from build123d import *

# Parameters (mm, degrees)
BOSS_EXTRUDE1_DEPTH = 2


with BuildPart() as part:
    # Sketch1 → Boss-Extrude1 (new body)
    with BuildSketch(Plane(origin=(0, 0, 0), x_dir=(0, 0, -1), z_dir=(1, 0, 0))):
        Polygon((20, 0), (0, 0), (0, 25), (-20, 25), (-20, 0), (-40, 0), (-40, -70), (20, -70), align=None)
        with BuildLine():
            ThreePointArc((9.318516526, -50.176380902), (-10, -65), (-29.318516526, -50.176380902))
            Line((-29.318516526, -50.176380902), (-32.5, -45))
            Line((-32.5, -45), (-32.5, -5))
            Line((-32.5, -5), (-20, -5))
            Line((-20, -5), (-20, -25))
            Line((-20, -25), (-17.5, -25))
            Line((-17.5, -25), (-15.75, -24.318465914))
            ThreePointArc((-15.75, -24.318465914), (-10, -22.5), (-4.25, -24.318465914))
            Line((-4.25, -24.318465914), (-2.5, -25))
            Line((-2.5, -25), (0, -25))
            Line((0, -25), (0, -4.981590289))
            Line((0, -4.981590289), (12.5, -5))
            Line((12.5, -5), (12.5, -45))
            Line((12.5, -45), (9.318516526, -50.176380902))
        make_face(mode=Mode.SUBTRACT)
    extrude(amount=BOSS_EXTRUDE1_DEPTH)


solid = part.part
Geometry: final body of the model. Coordinates: model frame, mm. A direction names the side the tool comes from. Coordinates: 2 decimals unless noted, no trailing zeros. Order: outer loops, then holes, each group sorted by start corner. A loop starts at its lowest first (then second) coordinate and runs counter-clockwise, first axis right, second up. Notation, with made-up numbers: (-28, -31.75) - (-9, -31.75) arc R16 ccw to (-9, -2.75) - close; hole circle Ø11 at (54.25, -6.75). An arc over 180 degrees is marked (long way). Use one line per item in the form item = value.
1) Set-up query: faces 5 (the face through (1, 13, 20)), 6 (the face through (1, 12, 0)), 7 (the face through (1, -25, 32.5)). Return all of +Z, -Z, +X, -X, +Y, -Y with unobstructed straight access to the full face (end or side cutting, diameter ignored); none if empty.
Solutions:
face_5 = +Z, +X, -X, +Y
face_6 = -Z, +X, -X, +Y
face_7 = +X, -X
2) Section B-B (y = -37). Return loops of the section in (x, z).
Solutions:
outline = (0, -20) - (2, -20) - (2, -12.5) - (0, -12.5) - close; (0, 32.5) - (2, 32.5) - (2, 40) - (0, 40) - close
3) Section A-A (y = -14). Return loops of the section in (x, z), then the cut area to 3 significant figures.
Solutions:
outline = (0, -20) - (2, -20) - (2, -12.5) - (0, -12.5) - close; (0, 0) - (2, 0) - (2, 20) - (0, 20) - close; (0, 32.5) - (2, 32.5) - (2, 40) - (0, 40) - close
area = 70.0 mm^2
4) Pin query (flat end, axial travel): pin 1 (0.6 mm diameter, centred on x = 1.5, z = -6, fed in from +Y); pin 2 (3 mm diameter, centred on y = 7.5, z = 18.5, fed in from -X); pin 3 (1 mm diameter, centred on x = 1, y = 13, fed in from -Z). Return the tip coordinate at first contact, or that it passes through.
Solutions:
pin_1 = 0
pin_2 = 0
pin_3 = 0
5) Section C-C (z = 5.5). Return loops of the section in (x, y).
Solutions:
outline = (0, -70) - (2, -70) - (2, -64.49) - (0, -64.49) - close; (0, -23.57) - (2, -23.57) - (2, 25) - (0, 25) - close
6) Section D-D (x = 0.4). Return loops of the section in (y, z), then the cut area to 3 significant figures.
Solutions:
outline = (-70, -20) - (0, -20) - (0, 0) - (25, 0) - (25, 20) - (0, 20) - (0, 40) - (-70, 40) - close; hole (-50.18, -9.32) - (-45, -12.5) - (-5, -12.5) - (-4.98, 0) - (-25, 0) - (-25, 2.5) - (-24.32, 4.25) arc R10 ccw to (-24.32, 15.75) - (-25, 17.5) - (-25, 20) - (-5, 20) - (-5, 32.5) - (-45, 32.5) - (-50.18, 29.32) arc R20 ccw to start
area = 2,640 mm^2
7) Mould query, pull axis Y, two halves, no side actions, for faces 1 (the face through (1, -5, 26)), 2 (the face through (0, -22, 10)), 3 (the face through (1, -70, 10)), 4 (the face through (1, 25, 10)). Classes: +Y half, -Y half, draft (parallel to the pull), parting line (faces both ways), or undercut.
Solutions:
face_1 = undercut
face_2 = draft
face_3 = -Y half
face_4 = +Y half
8) Ray query, L1, parallel to Z at x = 1.35, y = -14; L2, parallel to Y at x = 1.15, z = 33; L3, parallel to Z at x = 1.35, y = -29. Return the intervals inside material, ascending.
Solutions:
L1 = -20 to -12.5, 0 to 20, 32.5 to 40
L2 = -70 to 0
L3 = -20 to -12.5, 32.5 to 40
